from build123d import *

# Parameters (mm, degrees)
SKETCH1_W           = 60
SKETCH1_H           = 60
BOSS_EXTRUDE1_DEPTH = 1
SKETCH2_R           = 2
CUT_EXTRUDE1_DEPTH  = 2
SKETCH3_R           = 0.5
CUT_EXTRUDE2_DEPTH  = 2
CUT_EXTRUDE3_DEPTH  = 10


with BuildPart() as part:
    # Sketch1 → Boss-Extrude1 (new body)
    with BuildSketch(Plane(origin=(0, 0, 0), x_dir=(1, 0, 0), z_dir=(0, 1, 0))):
        Rectangle(SKETCH1_W, SKETCH1_H)
    extrude(amount=BOSS_EXTRUDE1_DEPTH)

    # Sketch2 → Cut-Extrude1 (cut, through all)
    with BuildSketch(Plane(origin=(0, 1, 0), x_dir=(1, 0, 0), z_dir=(0, 1, 0))):
        with Locations((-26, 26)):
            Circle(SKETCH2_R)
        with Locations((0, 26)):
            Circle(SKETCH2_R)
        with Locations((26, 26)):
            Circle(SKETCH2_R)
        with Locations((26, -26)):
            Circle(SKETCH2_R)
        with Locations((0, -26)):
            Circle(SKETCH2_R)
        with Locations((-26, -26)):
            Circle(SKETCH2_R)
    extrude(amount=-CUT_EXTRUDE1_DEPTH, mode=Mode.SUBTRACT)

    # Sketch3 → Cut-Extrude2 (cut, through all)
    with BuildSketch(Plane(origin=(0, 1, 0), x_dir=(1, 0, 0), z_dir=(0, 1, 0))):
        with Locations((10, 0)):
            Circle(SKETCH3_R)
        with Locations((-10, 0)):
            Circle(SKETCH3_R)
    extrude(amount=-CUT_EXTRUDE2_DEPTH, mode=Mode.SUBTRACT)

    # Sketch7 → Cut-Extrude3 (cut)
    with BuildSketch(Plane(origin=(0, 1, 0), x_dir=(1, 0, 0), z_dir=(0, 1, 0))):
        with BuildLine():
            add(Edge.make_bspline(
                [(10, 0.5), (7.54185609, 0.971550622), (5.54199885, 4.633621193), (0, 6.558338078), (-5.54199885, 4.633621193), (-7.54185609, 0.971550622), (-10, 0.5)],
                knots=[0, 0, 0, 0, 0.295686937, 0.5, 0.704313063, 1, 1, 1, 1], degree=3))
            add(Edge.make_bspline(
                [(-10, 0.5), (-11, 0), (-10, -0.5)],
                knots=[0, 0, 0, 1, 1, 1], degree=2))
            add(Edge.make_bspline(
                [(10, -0.5), (7.539614158, -0.960866701), (5.551451154, -4.662870645), (0, -6.482717161), (-5.551451154, -4.662870645), (-7.539614158, -0.960866701), (-10, -0.5)],
                knots=[0, 0, 0, 0, 0.296041393, 0.5, 0.703958607, 1, 1, 1, 1], degree=3))
            add(Edge.make_bspline(
                [(10, 0.5), (11, 0), (10, -0.5)],
                knots=[0, 0, 0, 1, 1, 1], degree=2))
        make_face()
    extrude(amount=-CUT_EXTRUDE3_DEPTH, mode=Mode.SUBTRACT)


solid = part.part
Verification items for the finished model (mm, model axes). Coordinates: 2 decimals unless noted, no trailing zeros. Order: outer loops, then holes, each group sorted by start corner. A loop starts at its lowest first (then second) coordinate and runs counter-clockwise, first axis right, second up.
1. Scan lines: line 1 (X direction, y = 0.25, z = -26); line 2 (Z direction, x = -26, y = 0.6); line 3 (X direction, y = 0.3, z = -25). Record each from-to range of solid material in increasing order.
Results found:
line 1: x = -30 to -28, -24 to -2, 2 to 24, 28 to 30
line 2: z = -30 to -28, -24 to 24, 28 to 30
line 3: x = -30 to -27.73, -24.27 to -1.73, 1.73 to 24.27, 27.73 to 30
2. Release check for a two-part mould opening along Z. For faces 1 (the face through (25.566, 0.507, 27.952)), 2 (the face through (0, 1, -7)), 3 (the face through (-26.434, 0.507, -24.048)) record: +Z half, -Z half, draft (parallel to the pull), parting line (faces both ways), or undercut.
Results found:
face 1: undercut
face 2: draft
face 3: undercut
3. Go/stop test with a flat-tipped pin: pin 1 Ø2.5 at (x, z) = (-26, 26) entering from -Y. Record where the tip stops, or that it passes through.
Results found:
pin 1: passes through
4. Sectioned sample at C-C, the plane y = 0.45. Give the number of separate pieces and of enclosed holes in the cut face, and give its area (3 significant figures).
Results found:
separate pieces: 1
enclosed holes: 7
area: 3,380 mm2
5. Sectioned sample at B-B, the plane x = -26. Record the cut outline in (y, z).
Results found:
outline: (0, -30) - (1, -30) - (1, -28) - (0, -28) - close; (0, -24) - (1, -24) - (1, 24) - (0, 24) - close; (0, 28) - (1, 28) - (1, 30) - (0, 30) - close
6. Sectioned sample at A-A, the plane z = -26. Record the cut outline in (x, y).
Results found:
outline: (-30, 0) - (-28, 0) - (-28, 1) - (-30, 1) - close; (-24, 0) - (-2, 0) - (-2, 1) - (-24, 1) - close; (2, 0) - (24, 0) - (24, 1) - (2, 1) - close; (28, 0) - (30, 0) - (30, 1) - (28, 1) - close
